Could you check a few things on this model? Use its own coordinates, in mm. A direction names the side the tool comes from. Round coordinates to 2 decimals unless told otherwise and drop trailing zeros. Loops run counter-clockwise (first coordinate to the right, second up) from the corner with the lowest first, then second, coordinate; pieces in that order, holes last. Notation, with made-up numbers: (11, 20) -> (29, 20) arc R27 ccw to (29, 59) -> close; hole circle Ø8 at (89, -36). An arc over 180 degrees is marked (long way). One line per item, written item: value.
```python
from build123d import *

# Parameters (mm, degrees)
SKETCH1_W           = 32.25
SKETCH1_H           = 20
SKETCH1_R           = 3.400367627
SKETCH1_H_2         = 24.25
SKETCH1_R_2         = 8.5
SKETCH1_R_3         = 4
BOSS_EXTRUDE1_DEPTH = 3.25
SKETCH1_3_W         = 32.25
SKETCH1_3_H         = 24.25
SKETCH1_3_R         = 8.5
BOSS_EXTRUDE2_DEPTH = 8.25
FILLET1_R           = 1


with BuildPart() as part:
    # Sketch1 → Boss-Extrude1 (new body)
    # profile 1 of 3: a face of its own
    with BuildSketch(Plane.XY):
        with Locations((16.125, 10)):
            Rectangle(SKETCH1_W, SKETCH1_H)
        with Locations(Location((6.125, 10, 0), (0, 0, 180))):
            Circle(SKETCH1_R, mode=Mode.SUBTRACT)
        with Locations(Location((26.125, 10, 0), (0, 0, 180))):
            Circle(SKETCH1_R, mode=Mode.SUBTRACT)
    # profile 2 of 3: a face of its own
    with BuildSketch(Plane.XY):
        with Locations((16.125, 32.125)):
            Rectangle(SKETCH1_W, SKETCH1_H_2)
        with Locations((16.125, 32.5)):
            Circle(SKETCH1_R_2, mode=Mode.SUBTRACT)
    # profile 3 of 3: a face of its own
    with BuildSketch(Plane.XY):
        with Locations((16.125, 32.5)):
            Circle(SKETCH1_R_2)
        with Locations(Location((16.125, 32.5, 0), (0, 0, 180))):
            Circle(SKETCH1_R_3, mode=Mode.SUBTRACT)
    extrude(amount=BOSS_EXTRUDE1_DEPTH)

    # Sketch1_3 → Boss-Extrude2 (add)
    with BuildSketch(Plane.XY):
        with Locations((16.125, 32.125)):
            Rectangle(SKETCH1_3_W, SKETCH1_3_H)
        with Locations((16.125, 32.5)):
            Circle(SKETCH1_3_R, mode=Mode.SUBTRACT)
    extrude(amount=BOSS_EXTRUDE2_DEPTH)

    # Fillet1
    fillet1_edges = [part.edges().sort_by_distance(p)[0] for p in [
        (16.125, 20, 3.25),
        (16.125, 20, 8.25),
    ]]
    fillet(fillet1_edges, radius=FILLET1_R)


solid = part.part
```
(1) Imagine slicing it at B-B on z = 1.5. Write out the boundary of the cut face in (x, y) (3 decimals), then the cut area to 3 significant figures.
Results below:
outline: (0, 0) -> (32.25, 0) -> (32.25, 44.25) -> (0, 44.25) -> close; hole circle Ø6.801 at (6.125, 10); hole circle Ø8 at (16.125, 32.5); hole circle Ø6.801 at (26.125, 10)
area: 1,300 mm²
(2) Imagine slicing it at C-C on x = 30. Write out the boundary of the cut face in (y, z).
Results below:
outline: (0, 0) -> (44.25, 0) -> (44.25, 8.25) -> (21, 8.25) arc R1 ccw to (20, 7.25) -> (20, 4.25) arc R1 cw to (19, 3.25) -> (0, 3.25) -> close
(3) Imagine slicing it at D-D on y = 32.5. Write out the boundary of the cut face in (x, z) (3 decimals).
Results below:
outline: (0, 0) -> (12.125, 0) -> (12.125, 3.25) -> (7.625, 3.25) -> (7.625, 8.25) -> (0, 8.25) -> close; (20.125, 0) -> (32.25, 0) -> (32.25, 8.25) -> (24.625, 8.25) -> (24.625, 3.25) -> (20.125, 3.25) -> close
(4) Please list where these lines run through material, in increasing order: L1, parallel to X at y = 10, z = 1.95; L2, parallel to X at y = 32.5, z = 1.8 (3 decimals); L3, parallel to Y at x = 16, z = 1.
Results below:
L1: x = 0 to 2.72, 9.53 to 22.72, 29.53 to 32.25
L2: x = 0 to 12.125, 20.125 to 32.25
L3: y = 0 to 28.5, 36.5 to 44.25
(5) On a 3-axis mill with a long thin cutter (end or side, diameter ignored), from which of +Z, -Z, +X, -X, +Y, -Y can I reach the whole of each face in a straight line? I mean faces 1 (the face through (16, 22, 0)), 2 (the face through (16, 10, 3.25)), 3 (the face through (20, 31, 3.25)). Say none if no direction works.
Results below:
face 1: -Z, +X, -X, +Y, -Y
face 2: +Z, +X, -X, -Y
face 3: +Z
(6) Imagine slicing it at A-A on y = 10. Write out the boundary of the cut face in (x, z), then the cut area to 3 significant figures.
Results below:
outline: (0, 0) -> (2.72, 0) -> (2.72, 3.25) -> (0, 3.25) -> close; (9.53, 0) -> (22.72, 0) -> (22.72, 3.25) -> (9.53, 3.25) -> close; (29.53, 0) -> (32.25, 0) -> (32.25, 3.25) -> (29.53, 3.25) -> close
area: 60.6 mm²
(7) We'd pull the mould along X, two halves only. Please class faces 4 (the face through (0, 27, 3)), 5 (the face through (16, 44.25, 4)), 6 (the face through (22.984, 11.302, 1.602)): +X half, -X half, draft (parallel to the pull), parting line (faces both ways), or undercut.
Results below:
face 4: -X half
face 5: draft
face 6: undercut
(8) For pin 1 Ø4 at (x, z) = (24.5, 4) entering from -Y; pin 2 Ø10.5 at (x, y) = (16.125, 32.5) entering from +Z; pin 3 Ø4 at (x, y) = (6.125, 10) entering from +Z; pin 4 Ø3.5 at (x, z) = (18, 6) entering from -Y, each with a flat end and sliding along its axis, tell me the tip position at first contact or that it passes through.
Results below:
pin 1: stops at y = 0
pin 2: stops at z = 3.25
pin 3: passes through
pin 4: stops at y = 20
